Read the model definition and answer for the solid it produces. Units are mm, in the model's axes. A direction names the side the tool comes from. Round coordinates to 2 decimals unless told otherwise and drop trailing zeros. Write each loop counter-clockwise with the first axis right and the second up, starting at its lowest first coordinate (ties: lowest second). Pieces come first, ordered by that corner, then holes.
from build123d import *

# Parameters (mm, degrees)
SKETCH1_W           = 104.14
SKETCH1_H           = 102.87
SKETCH1_R           = 1.524
BOSS_EXTRUDE1_DEPTH = 1.778
SKETCH2_W           = 57.912
SKETCH2_H           = 8.636
SKETCH2_W_2         = 15.9512
SKETCH2_H_2         = 12
SKETCH2_W_3         = 30.988
SKETCH2_H_3         = 15.24
SKETCH2_W_4         = 86.106
SKETCH2_H_4         = 6.858
SKETCH2_W_5         = 6.858
SKETCH2_H_5         = 30.988
SKETCH2_H_6         = 7.62
BOSS_EXTRUDE2_DEPTH = 11.303
SKETCH3_W           = 11.938
SKETCH3_H           = 32.58
SKETCH3_W_2         = 3.81
SKETCH3_H_2         = 7.366
BOSS_EXTRUDE3_DEPTH = 7.62
SKETCH4_R           = 1.74625
BOSS_EXTRUDE4_DEPTH = 0.762
SKETCH5_W           = 22.606
SKETCH5_H           = 1.778
BOSS_EXTRUDE5_DEPTH = 27.432


with BuildPart() as part:
    # Sketch1 → Boss-Extrude1 (new body)
    with BuildSketch(Plane.XY):
        Rectangle(SKETCH1_W, SKETCH1_H)
        with Locations((-48.26, 47.625)):
            Circle(SKETCH1_R, mode=Mode.SUBTRACT)
        with Locations((48.26, 47.625)):
            Circle(SKETCH1_R, mode=Mode.SUBTRACT)
        with Locations((48.26, -47.625)):
            Circle(SKETCH1_R, mode=Mode.SUBTRACT)
        with Locations((-48.26, -47.625)):
            Circle(SKETCH1_R, mode=Mode.SUBTRACT)
    extrude(amount=BOSS_EXTRUDE1_DEPTH)

    # Sketch2 → Boss-Extrude2 (add)
    with BuildSketch(Plane.XY.offset(1.778)):
        with Locations((-14.224, 43.307)):
            Rectangle(SKETCH2_W, SKETCH2_H)
        with Locations((-47.9044, 6.955)):
            Rectangle(SKETCH2_W_2, SKETCH2_H_2)
        with Locations((-35.814, -12.065)):
            Rectangle(SKETCH2_W_3, SKETCH2_H_3)
        with Locations((-0.127, -45.466)):
            Rectangle(SKETCH2_W_4, SKETCH2_H_4)
        with Locations((36.449, -4.699)):
            Rectangle(SKETCH2_W_5, SKETCH2_H_5)
        with Locations((24.257, 6.985)):
            Rectangle(SKETCH2_W_5, SKETCH2_H_6)
    extrude(amount=BOSS_EXTRUDE2_DEPTH)

    # Sketch3 → Boss-Extrude3 (add)
    with BuildSketch(Plane.XY.offset(1.778)):
        with Locations((47.625, 22.195)):
            Rectangle(SKETCH3_W, SKETCH3_H)
        with Locations((-50.165, 28.135)):
            Rectangle(SKETCH3_W_2, SKETCH3_H_2)
    extrude(amount=BOSS_EXTRUDE3_DEPTH)

    # Sketch4 → Boss-Extrude4 (add)
    with BuildSketch(Plane.ZY.offset(52.07)):
        with Locations(Location((6.096, 28.135, 0), (0, 0, 90))):  # turned: the seam where the file's is
            Circle(SKETCH4_R)
    extrude(amount=BOSS_EXTRUDE4_DEPTH)

    # Sketch5 → Boss-Extrude5 (add)
    with BuildSketch(Plane.XY.offset(1.778)):
        with Locations((31.623, 40.894)):
            Rectangle(SKETCH5_W, SKETCH5_H)
    extrude(amount=BOSS_EXTRUDE5_DEPTH)


solid = part.part
Q1. Section A-A (x = 48.26) is taken. Determine the outline of the cut face in (y, z) (3 decimals).
Verdict:
outline: (-51.435, 0) - (-49.149, 0) - (-49.149, 1.778) - (-51.435, 1.778) - close; (-46.101, 0) - (46.101, 0) - (46.101, 1.778) - (38.485, 1.778) - (38.485, 9.398) - (5.905, 9.398) - (5.905, 1.778) - (-46.101, 1.778) - close; (49.149, 0) - (51.435, 0) - (51.435, 1.778) - (49.149, 1.778) - close
Q2. Section C-C (y = -7) is taken. Determine the outline of the cut face in (x, z), then the cut area to 3 significant figures.
Verdict:
outline: (-52.07, 0) - (52.07, 0) - (52.07, 1.78) - (39.88, 1.78) - (39.88, 13.08) - (33.02, 13.08) - (33.02, 1.78) - (-20.32, 1.78) - (-20.32, 13.08) - (-51.31, 13.08) - (-51.31, 1.78) - (-52.07, 1.78) - close
area: 613 mm2
Q3. Determine the mould class of faces 6 (the flat face through (-52.832, 28, 6)), 7 (the flat face through (-48, 7, 13.081)), 8 (the cylindrical face through (49.668, 47.041, 0.877)), 9 (the flat face through (53.594, 22, 6)) for opening direction X: pulls with the +X half, pulls with the -X half, needs draft (parallel to the pull), parting line crosses it, or undercut.
Verdict:
face 6: pulls with the -X half
face 7: needs draft
face 8: undercut
face 9: pulls with the +X half
Q4. Section D-D (z = 15.5) is taken. Determine the outline of the cut face in (x, y) (3 decimals).
Verdict:
outline: (20.32, 40.005) - (42.926, 40.005) - (42.926, 41.783) - (20.32, 41.783) - close
Q5. Section B-B (x = 11.5) is taken. Determine the outline of the cut face in (y, z) (3 decimals).
Verdict:
outline: (-51.435, 0) - (51.435, 0) - (51.435, 1.778) - (47.625, 1.778) - (47.625, 13.081) - (38.989, 13.081) - (38.989, 1.778) - (-42.037, 1.778) - (-42.037, 13.081) - (-48.895, 13.081) - (-48.895, 1.778) - (-51.435, 1.778) - close
Q6. Flat-ended cylindrical pins translate along their axes: pin 1 Ø2 at (x, y) = (25, 5.5) entering from +Z; pin 2 Ø7.5 at (x, z) = (35, 8) entering from +Y; pin 3 Ø10 at (y, z) = (-8.5, 4) entering from -X. Find the tip coordinate at first contact, or state that the pin passes through.
Verdict:
pin 1: stops at z = 13.08
pin 2: stops at y = 41.78
pin 3: stops at x = -52.07
Q7. Which of the six approach directions +Z, -Z, +X, -X, +Y, -Y give full straight-line access (tool end or side, diameter ignored) to faces 1 (the flat face through (-54, 7, 1.778)), 2 (the flat face through (36, -4, 13.081)), 3 (the flat face through (-48, 0.955, 7)), 4 (the flat face through (31, 40.005, 15)), 5 (the flat face through (31, 41.783, 15))?
Verdict:
face 1: -Z, -X, +Y, -Y
face 2: +Z, +X, -X, -Y
face 3: +Z, -X
face 4: +Z, +X
face 5: +Z, +X, +Y
Q8. Straight lines are drawn through the part: probe 1 along Y at (x, z) = (-48.26, 1) (3 decimals); probe 2 along X at (y, z) = (41.5, 4.5); probe 3 along Y at (x, z) = (26.5, 5.75) (3 decimals). For each, find the intervals that lie inside material, in ascending order.
Verdict:
probe 1: y = -51.435 to -49.149, -46.101 to 46.101, 49.149 to 51.435
probe 2: x = -43.18 to 14.73, 20.32 to 42.93
probe 3: y = -48.895 to -42.037, 3.175 to 10.795, 40.005 to 41.783
